from build123d import *

# Parameters (mm, degrees)
ESBO_O1_R                = 3
RESSALTO_EXTRUS_O1_DEPTH = 10
ESBO_O2_R                = 3
CORTE_EXTRUS_O1_DEPTH    = 10
CORTE_EXTRUS_O2_START    = -80
ESBO_O2_2_R              = 3
CORTE_EXTRUS_O2_DEPTH    = 10
FILETE1_R                = 3
ESBO_O3_W                = 90
ESBO_O3_H                = 2.5
RESSALTO_EXTRUS_O2_DEPTH = 10
ESBO_O4_W                = 2
ESBO_O4_H                = 5
CORTE_EXTRUS_O3_DEPTH    = 10
PADR_O_LINEAR1_COUNT     = 4
PADR_O_LINEAR1_PITCH     = 20


with BuildPart() as part:
    # Esboço1 → Ressalto-extrusão1 (new body)
    with BuildSketch(Plane(origin=(0, 0, 0), x_dir=(0, 0, -1), z_dir=(1, 0, 0))):
        with BuildLine():
            Line((15, 44), (0, 44))
            Line((0, 44), (0, 12))
            Line((0, 12), (-20, 12))
            Line((-20, 12), (-20, 0))
            Line((-20, 0), (70, 0))
            Line((70, 0), (70, 12))
            Line((70, 12), (55, 12))
            Line((55, 12), (55, 7.43))
            Line((55, 7.43), (12, 7.43))
            ThreePointArc((12, 7.43), (7.765686518, 4.695686516), (7.015686515, 9.679999999))
            Line((7.015686515, 9.679999999), (9, 11.430000002))
            Line((9, 11.430000002), (9, 34))
            Line((9, 34), (15, 34))
            Line((15, 34), (15, 44))
        make_face()
        with Locations((9, 39)):
            Circle(ESBO_O1_R, mode=Mode.SUBTRACT)
    extrude(amount=RESSALTO_EXTRUS_O1_DEPTH)

    # Esboço2 → Corte-extrusão1 (cut)
    with BuildSketch(Plane(origin=(0, 0, -70), x_dir=(-1, 0, 0), z_dir=(0, 0, -1))):
        with Locations((-5, 6)):
            Circle(ESBO_O2_R)
    extrude(amount=-CORTE_EXTRUS_O1_DEPTH, mode=Mode.SUBTRACT)

    # Esboço2<2> → Corte-extrusão2 (cut)
    with BuildSketch(Plane(origin=(0, 0, -70), x_dir=(-1, 0, 0), z_dir=(0, 0, -1)).offset(CORTE_EXTRUS_O2_START)):
        with Locations((-5, 6)):
            Circle(ESBO_O2_2_R)
    extrude(amount=-CORTE_EXTRUS_O2_DEPTH, mode=Mode.SUBTRACT)

    # Filete1
    filete1_edges = [part.edges().sort_by_distance(p)[0] for p in [
        (5, 7.43, -55),
        (5, 44, 0),
        (5, 44, -15),
        (5, 34, -15),
        (5, 34, -9),
    ]]
    fillet(filete1_edges, radius=FILETE1_R - 0.0001)  # a hair under: the kernel refuses the full size

    # Esboço3 → Ressalto-extrusão2 (add)
    with BuildSketch(Plane.ZY):
        with Locations((-25, 1.25)):
            Rectangle(ESBO_O3_W, ESBO_O3_H)
    extrude(amount=RESSALTO_EXTRUS_O2_DEPTH)

    # Esboço4 → Corte-extrusão3 (cut)
    with BuildSketch(Plane(origin=(0, 2.5, 0), x_dir=(1, 0, 0), z_dir=(0, 1, 0))):
        with Locations((-5, 57.5)):
            Rectangle(ESBO_O4_W, ESBO_O4_H)
    corte_extrus_o3 = extrude(amount=-CORTE_EXTRUS_O3_DEPTH, mode=Mode.SUBTRACT)

    # Padrão linear1: Corte-extrusão3 ×4
    with Locations(*[(0, 0, i * PADR_O_LINEAR1_PITCH) for i in range(1, PADR_O_LINEAR1_COUNT)]):
        add(corte_extrus_o3, mode=Mode.SUBTRACT)


solid = part.part
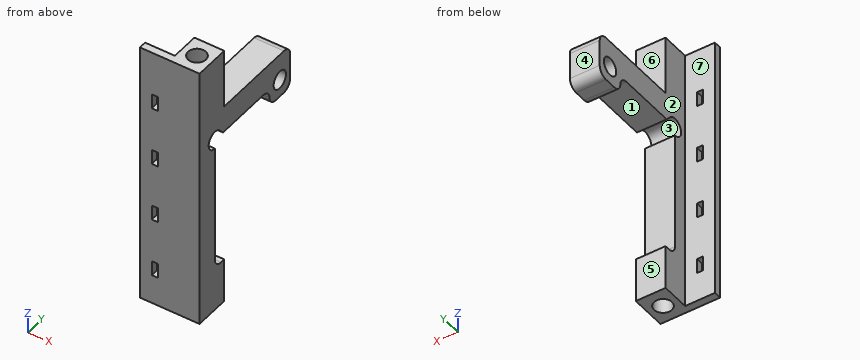
Part model, mm, in its own coordinate system. Face numbers are marked on the shaded views. A direction names the side the tool comes from. Give positions to 0.01 mm unless a question says otherwise; leave off trailing zeros. Order: outer loops, then holes, each group sorted by start corner. A loop starts at its lowest first (then second) coordinate and runs counter-clockwise, first axis right, second up. Notation, with made-up numbers: (-5, 76.25) - (34, 76.25) arc R22 cw to (34, 94.25) - close; hole circle Ø2 at (86.25, 47.5). An arc over 180 degrees is marked (long way). One line per question, with ' | ' between items.
1. Drop flat-ended pins along their axis: P1, Ø3, axis at x = 7, y = 33, coming from the +Z side; P2, Ø5.5, axis at y = 39, z = -9, coming from the -X side; P3, Ø12, axis at x = 1.5, y = 14.5, coming from the +Z side; P4, Ø1.2, axis at x = 7.5, y = 38.5, coming from the -Z side. Give the stop position or say it passes through.
Filled in:
P1: z = 0 | P2: through | P3: z = 20 | P4: z = -15
2. Band-saw the part on C-C on y = 39. List the corners of the cut face in (x, z).
Filled in:
outline: (0, -15) - (10, -15) - (10, -12) - (0, -12) - close; (0, -6) - (10, -6) - (10, 0) - (0, 0) - close
3. Band-saw the part on A-A on z = -18. List the corners of the cut face in (x, y), then the cut area to 3 significant figures.
Filled in:
outline: (-10, 0) - (-6, 0) - (-6, 2.5) - (-10, 2.5) - close; (-4, 0) - (10, 0) - (10, 7.43) - (0, 7.43) - (0, 2.5) - (-4, 2.5) - close | area: 94.3 mm²
4. Drill centre lines: probe 1 along Y at (x, z) = (5, 12.5); probe 2 along Y at (x, z) = (-6.5, 12.5); probe 3 along Y at (x, z) = (1.5, -51). Where is each one in solid material? Low to high.
Filled in:
probe 1: 0 to 3, 9 to 12 | probe 2: 0 to 2.5 | probe 3: 0 to 7.43
5. Which spindle directions (+Z, -Z, +X, -X, +Y, -Y) get a long thin tool onto all of the face, cutting with end or side? Do the marked faces 5, 6 and 7. Say none if no direction does.
Filled in:
face 5: -Z, +X, -X, +Y | face 6: +Z, +X, -X, +Y | face 7: +Z, -Z, -X, +Y
6. Band-saw the part on D-D on z = 14. List the corners of the cut face in (x, y).
Filled in:
outline: (-10, 0) - (10, 0) - (10, 12) - (0, 12) - (0, 2.5) - (-10, 2.5) - close; hole circle Ø6 at (5, 6)
7. Pull direction Y, two halves, no side cores. Call the marked faces 1, 2, 3 and 4: +Y half, -Y half, draft (parallel to the pull), parting line (faces both ways), or undercut.
Filled in:
face 1: undercut | face 2: draft | face 3: undercut | face 4: +Y half
